```python
from build123d import *

# Parameters (mm, degrees)
BOX_W               = 10
BOX_H               = 10
BOX_DEPTH           = 30
CYLINDER_R          = 2.6
CYLINDER_DEPTH      = 22
CUT_PLACEMENT_ANGLE = 45


with BuildPart() as cube:
    # Box → Box (new body)
    with BuildSketch(Plane(origin=(-5, 2, -1), x_dir=(1, 0, 0), z_dir=(0, 0, 1))):
        with Locations((5, 5)):
            Rectangle(BOX_W, BOX_H)
    extrude(amount=BOX_DEPTH)


with BuildPart() as motor_shaft:
    # Cylinder → Cylinder (new body)
    with BuildSketch(Plane.XY):
        Circle(CYLINDER_R)
    extrude(amount=CYLINDER_DEPTH)

    # Cut: cut Cube
    add(cube.part, mode=Mode.SUBTRACT)


with BuildPart() as motor_shaft_1:
    # Cut placement: moved
    add(motor_shaft.part.rotate(Axis((0, 0, 0), (0, 0, 1)), CUT_PLACEMENT_ANGLE))


solid = motor_shaft_1.part
```
Read the model definition and answer for the solid it produces. Units are mm, in the model's axes. Coordinates: 2 decimals unless noted, no trailing zeros. Write each loop counter-clockwise with the first axis right and the second up, starting at its lowest first coordinate (ties: lowest second). Pieces come first, ordered by that corner, then holes. Notation, with made-up numbers: (50, -34) -> (64, -34) arc R22 ccw to (64, -23) -> close; hole circle Ø4 at (-36, 68.25). An arc over 180 degrees is marked (long way). Answer as a JSON object with one key per item and string values.
Q1. Determine the mould class of faces 1 (the cylindrical face through (1.774, -1.9, 10.846)), 2 (the flat face through (0, 0, 22)), 3 (the flat face through (-1.43, 1.4, 10.85)) for opening direction X: pulls with the +X half, pulls with the -X half, needs draft (parallel to the pull), parting line crosses it, or undercut.
The answers:
{"face 1": "parting line crosses it", "face 2": "needs draft", "face 3": "pulls with the -X half"}
Q2. The part is cut by section A-A on z = 4.5. Give the vertices of the cut face in (x, y).
The answers:
{"outline": "(-2.59, 0.24) arc R2.6 ccw (long way) to (-0.24, 2.59) -> close"}
Q3. Consider line 1 (X direction, y = -0.25, z = 11.75); line 2 (Y direction, x = -0.4, z = 4.25). Determine where each line is inside the solid, lowest interval first. Write a range as [from, to].
The answers:
{"line 1": "x = [-2.59, 2.59]", "line 2": "y = [-2.57, 2.43]"}
Q4. The part is cut by section C-C on x = 1.45. Give the vertices of the cut face in (y, z).
The answers:
{"outline": "(-2.16, 0) -> (2.16, 0) -> (2.16, 22) -> (-2.16, 22) -> close"}
Q5. The part is cut by section B-B on y = 2.25. Give the vertices of the cut face in (x, z), then the cut area to 3 significant figures.
The answers:
{"outline": "(-0.58, 0) -> (1.3, 0) -> (1.3, 22) -> (-0.58, 22) -> close", "area": "41.4 mm2"}
Q6. Flat-ended cylindrical pins translate along their axes: pin 1 Ø1.5 at (x, z) = (1, 7.5) entering from -Y; pin 2 Ø1 at (x, z) = (-1.5, 9) entering from -Y; pin 3 Ø2 at (y, z) = (1.5, 10.5) entering from +X. Find the tip coordinate at first contact, or state that the pin passes through.
The answers:
{"pin 1": "stops at y = -2.59", "pin 2": "stops at y = -2.4", "pin 3": "stops at x = 2.55"}
